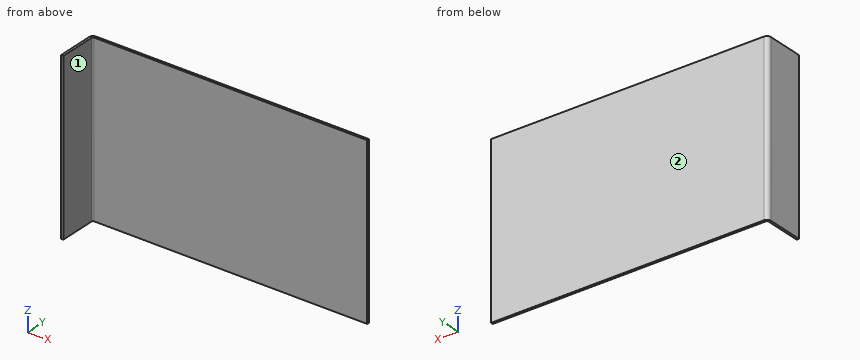
```python
from build123d import *

# Parameters (mm, degrees)
SKETCH_1_W                       = 180
SKETCH_1_H                       = 109
SM_BASE_FLANGE_1_DEPTH           = 1.5
SM_EDGE_FLANGE_1_STRIP_W         = 8
SM_EDGE_FLANGE_1_STRIP_H         = 1.5
SM_EDGE_FLANGE_1_STRIP_CUT_DEPTH = 109
SM_EDGE_FLANGE_1_DEPTH           = 109


# Sheet-metal steps are written as plain solids
with BuildPart() as part:
    # Sketch 1 → 基体-法兰1 (new body)
    with BuildSketch(Plane(origin=(0, 0, 0), x_dir=(1, 0, 0), z_dir=(0, 1, 0))):
        Rectangle(SKETCH_1_W, SKETCH_1_H)
    extrude(amount=-SM_BASE_FLANGE_1_DEPTH)

    # 边线-法兰1 strip (across the edge) → 边线-法兰1 strip cut (cut)
    with BuildSketch(Plane(origin=(-90, -1.5, 54.5), x_dir=(1, 0, 0), z_dir=(0, 0, -1))):
        with Locations((-1.5, -0.75)):
            Rectangle(SM_EDGE_FLANGE_1_STRIP_W, SM_EDGE_FLANGE_1_STRIP_H)
    extrude(amount=SM_EDGE_FLANGE_1_STRIP_CUT_DEPTH, mode=Mode.SUBTRACT)

    # 边线-法兰1 section (across the edge) → 边线-法兰1 (add)
    with BuildSketch(Plane(origin=(-90, -1.5, 54.5), x_dir=(1, 0, 0), z_dir=(0, 0, -1))):
        with BuildLine():
            Line((0, 1), (0, 25))
            Line((0, 25), (1.5, 25))
            Line((1.5, 25), (1.5, 1))
            ThreePointArc((1.5, 1), (1.792893219, 0.292893219), (2.5, 0))
            Line((2.5, 0), (2.5, -1.5))
            ThreePointArc((2.5, -1.5), (0.732233047, -0.767766953), (0, 1))
        make_face()
    extrude(amount=SM_EDGE_FLANGE_1_DEPTH)


solid = part.part
```
The model under review builds one solid part; all positions refer to its coordinate system, in mm. Face numbers are marked on the shaded views. A direction names the side the tool comes from. Round coordinates to 2 decimals unless told otherwise and drop trailing zeros. Write each loop counter-clockwise with the first axis right and the second up, starting at its lowest first coordinate (ties: lowest second). Pieces come first, ordered by that corner, then holes. Notation, with made-up numbers: (75.5, 30) - (99.5, 30) arc R23 cw to (99.5, 38) - close; hole circle Ø6 at (-4, -15.5). An arc over 180 degrees is marked (long way). Answer as CSV lines item,"result". Start each with the question number.
(1) To check wall thickness, follow line 1 (X direction, y = -10.25, z = -40); line 2 (Y direction, x = -13, z = 13); line 3 (X direction, y = -1, z = 16.5). State the ranges of each line that lie inside material, in increasing order.
(2) For the marked faces 1 and 2, list the 3-axis set-ups (+Z, -Z, +X, -X, +Y, -Y) from which the entire face can be reached by the end or side of a thin tool; tool diameter is ignored.
(3) We need section C-C on y = -6.25. State the section outline as (x, z) points.
(4) For pin 1 Ø1.5 at (y, z) = (-6, 25.5) entering from +X; pin 2 Ø4 at (x, z) = (69.5, 16) entering from -Y, all flat-tipped, find the tip position at first contact; note any pin that passes through.
(5) We need section B-B on x = -60.5. State the section outline as (y, z) points, plus the area to 4 significant figures.
(6) We need section A-A on z = -18. State the section outline as (x, y) points, plus the area to 3 significant figures.
Worked answers:
1,line 1,"-90 to -88.5"
1,line 2,"-1.5 to 0"
1,line 3,"-89.5 to 90"
2,face 1,"+Z, -Z, +X, -Y"
2,face 2,"+Z, -Z, +X, -X, +Y"
3,outline,"(-90, -54.5) - (-88.5, -54.5) - (-88.5, 54.5) - (-90, 54.5) - close"
4,pin 1,"x = -88.5"
4,pin 2,"y = -1.5"
5,outline,"(-1.5, -54.5) - (0, -54.5) - (0, 54.5) - (-1.5, 54.5) - close"
5,area,"163.5 mm²"
6,outline,"(-90, -26.5) - (-88.5, -26.5) - (-88.5, -2.5) arc R1 cw to (-87.5, -1.5) - (90, -1.5) - (90, 0) - (-87.5, 0) arc R2.5 ccw to (-90, -2.5) - close"
6,area,"306 mm²"
